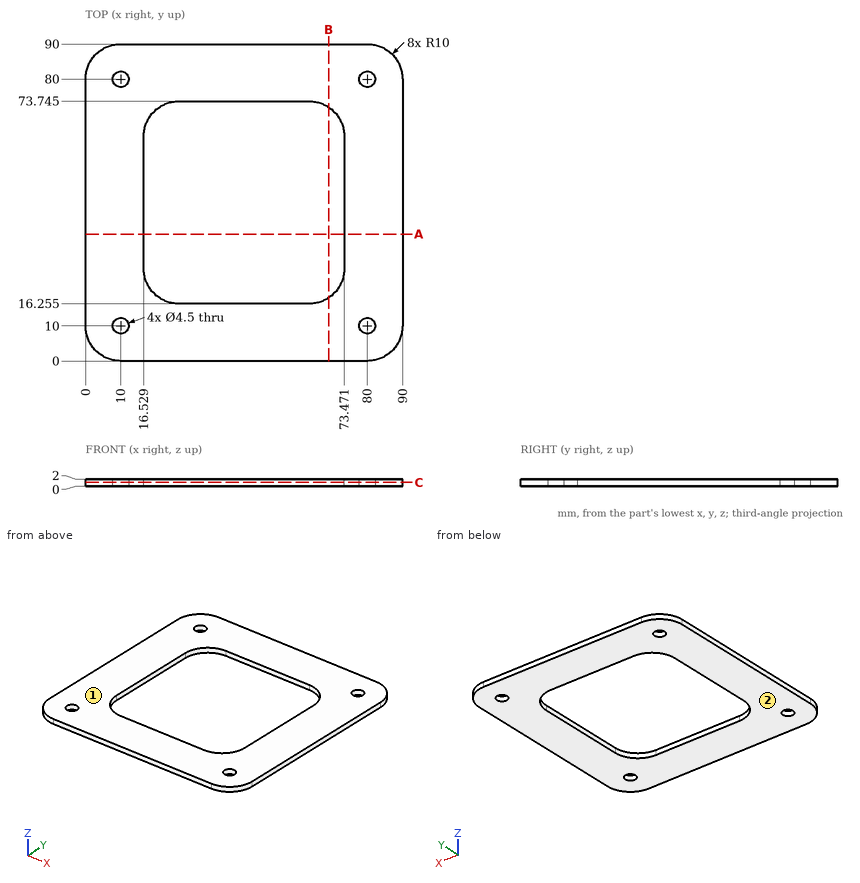
Source: three-view drawing plus pictorial views. Frame: mm from the lowest corner of the part. Round coordinates to 2 decimals unless told otherwise and drop trailing zeros. Order: outer loops, then holes, each group sorted by start corner. A loop starts at its lowest first (then second) coordinate and runs counter-clockwise, first axis right, second up. Notation, with made-up numbers: (87.25, 9.25) -> (138.25, 9.25) arc R20 cw to (138.25, 35.25) -> close; hole circle Ø2 at (66, -37). An arc over 180 degrees is marked (long way). Use one line per item in the form item = value. Start each with the question number.
1. Line query: probe 1 along Y at (x, z) = (80, 1.4); probe 2 along Y at (x, z) = (26, 0.3). Output: solid intervals per line, ascending.
2. Cut plane C-C (z = 1.05). Count the separate pieces of the cut face and the enclosed holes in it, then the cut area to 3 significant figures.
3. Cut plane A-A (y = 36). Return the cut outline in (x, z).
4. Draft query along Z for the marked faces 1 and 2. Return one class per face: pulls with the +Z half, pulls with the -Z half, needs draft (parallel to the pull), parting line crosses it, or undercut.
5. Cut plane B-B (x = 69). Return the cut outline in (y, z).
Solution:
q1.probe_1 = 0 to 7.75, 12.25 to 77.75, 82.25 to 90
q1.probe_2 = 0 to 16.27, 73.73 to 90
q2.separate_pieces = 1
q2.enclosed_holes = 5
q2.area = 4,760 mm^2
q3.outline = (0, 0) -> (16.53, 0) -> (16.53, 2) -> (0, 2) -> close; (73.47, 0) -> (90, 0) -> (90, 2) -> (73.47, 2) -> close
q4.face_1 = pulls with the +Z half
q4.face_2 = pulls with the -Z half
q5.outline = (0, 0) -> (17.92, 0) -> (17.92, 2) -> (0, 2) -> close; (72.08, 0) -> (90, 0) -> (90, 2) -> (72.08, 2) -> close
